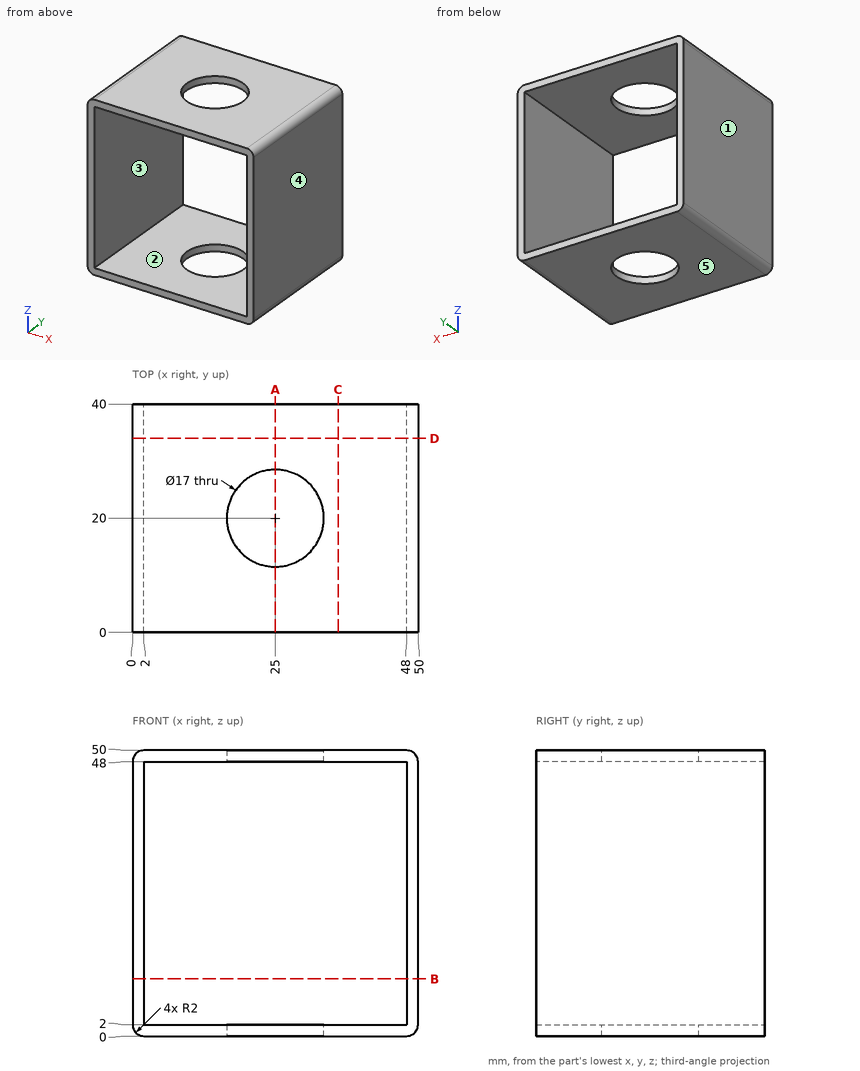
Can you work these out from the drawing? Everything is in mm from the part's minimum corner. A direction names the side the tool comes from. Round coordinates to 2 decimals unless told otherwise and drop trailing zeros. Loops run counter-clockwise (first coordinate to the right, second up) from the corner with the lowest first, then second, coordinate; pieces in that order, holes last.
1. If we section it at C-C on x = 36: Write out the boundary of the cut face in (y, z).
Answer list:
outline: (0, 0) - (40, 0) - (40, 2) - (0, 2) - close; (0, 48) - (40, 48) - (40, 50) - (0, 50) - close
2. Which directions (+Z, -Z, +X, -X, +Y, -Y) give clear straight access to the entire face, cutting with the end or side of a thin tool? Please do the marked faces 1 and 2.
Answer list:
face 1: +Z, -Z, -X, +Y, -Y
face 2: +Y, -Y
3. We'd pull the mould along Z, two halves only. Please class the marked faces 3, 4 and 5: +Z half, -Z half, draft (parallel to the pull), parting line (faces both ways), or undercut.
Answer list:
face 3: undercut
face 4: draft
face 5: -Z half
4. If we section it at D-D on y = 34: Write out the boundary of the cut face in (x, z).
Answer list:
outline: (0, 2) arc R2 ccw to (2, 0) - (48, 0) arc R2 ccw to (50, 2) - (50, 48) arc R2 ccw to (48, 50) - (2, 50) arc R2 ccw to (0, 48) - close; hole (2, 2) - (48, 2) - (48, 48) - (2, 48) - close
5. If we section it at A-A on x = 25: Write out the boundary of the cut face in (y, z), plus the area to 3 significant figures.
Answer list:
outline: (0, 0) - (11.5, 0) - (11.5, 2) - (0, 2) - close; (0, 48) - (11.5, 48) - (11.5, 50) - (0, 50) - close; (28.5, 0) - (40, 0) - (40, 2) - (28.5, 2) - close; (28.5, 48) - (40, 48) - (40, 50) - (28.5, 50) - close
area: 92.0 mm2
6. If we section it at B-B on z = 10: Write out the boundary of the cut face in (x, y).
Answer list:
outline: (0, 0) - (2, 0) - (2, 40) - (0, 40) - close; (48, 0) - (50, 0) - (50, 40) - (48, 40) - close
7. If I drill on line 1 along Z through (x, y) = (21, 6); line 2 along Y through (x, z) = (25, 0.6), over which ranges is the centre line in solid material (lowest first)?
Answer list:
line 1: z = 0 to 2, 48 to 50
line 2: y = 0 to 11.5, 28.5 to 40
